Geometry: final body of the model. Coordinates: model frame, mm. Face numbers are marked on the shaded views. Round coordinates to 2 decimals unless told otherwise and drop trailing zeros. Write each loop counter-clockwise with the first axis right and the second up, starting at its lowest first coordinate (ties: lowest second). Pieces come first, ordered by that corner, then holes. Notation, with made-up numbers: M 51,-1 L 79,-1 A12 ccw 79,5 Z; hole C 86,58 d2. An arc over 180 degrees is marked long. Answer as CSV lines item,"result". Start each with the question number.
Q1. First-contact query: pin 1 (5 mm diameter, centred on x = 6.5, y = 4.5, fed in from +Z); pin 2 (2 mm diameter, centred on x = -8, z = 3.5, fed in from +Y); pin 3 (1 mm diameter, centred on x = 11, z = 2, fed in from -Y). Flat tips, straight axial feed; report the tip coordinate or a pass-through.
Q2. Section query A-A on z = 3.25. Output: boundary loops of the cut face in (x, y).
Q3. Section query B-B on x = -9. Output: boundary loops of the cut face in (y, z).
Q4. Ray query, probe 1 along Y at (x, z) = (3.5, 1.2); probe 2 along X at (y, z) = (1.5, 0.55); probe 3 along Z at (x, y) = (9, -1). Return the intervals inside material, ascending.
Q5. Mould query, pull axis X, two halves, no side actions, for the marked faces 1, 2, 3 and 4. Classes: pulls with the +X half, pulls with the -X half, needs draft (parallel to the pull), parting line crosses it, or undercut.
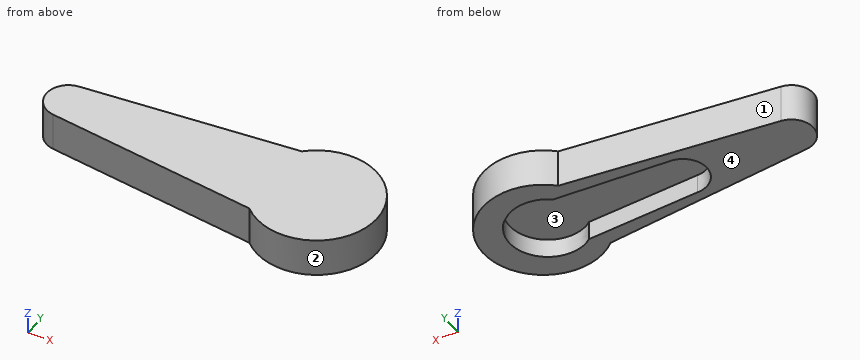
```python
from build123d import *

# Parameters (mm, degrees)
BOSS_EXTRUDE6_DEPTH = 4
CUT_EXTRUDE1_DEPTH  = 2


with BuildPart() as part:
    # Sketch2 → Boss-Extrude6 (new body)
    with BuildSketch(Plane.XY):
        with BuildLine():
            Line((7.936945185, 4.607509822), (-13.764834635, 2.265131203))
            ThreePointArc((-13.764834635, 2.265131203), (-15.798635322, 0), (-13.764834635, -2.265131203))
            Line((-13.764834635, -2.265131203), (7.936945185, -4.607509822))
            ThreePointArc((7.936945185, -4.607509822), (18.479455181, 0), (7.936945185, 4.607509822))
        make_face()
    extrude(amount=BOSS_EXTRUDE6_DEPTH)

    # Sketch1 → Cut-Extrude1 (cut)
    with BuildSketch(Plane.XY):
        with BuildLine():
            Line((-2.308259951, 2.498066053), (9.375044145, 3.190055955))
            add(Edge.make_bspline(
                [(9.375044145, 3.190055955), (9.743762717, 3.535051607), (10.542113364, 3.885379294), (11.739855888, 4.053778423), (12.781606273, 3.904003548), (13.647647588, 3.58835165), (14.172524986, 3.123610305), (14.749448402, 2.727996587), (15.239395752, 2.01553181), (15.653528757, 1.050879588), (15.788992815, -0.000691818), (15.651665108, -1.048112313), (15.246850359, -2.025217286), (14.603250264, -2.863967716), (13.764299096, -3.507779486), (12.787785525, -3.91194775), (11.73820132, -4.051651269), (10.542857019, -3.886335356), (9.743600409, -3.534842939), (9.375044145, -3.190055955)],
                knots=[0, 0, 0, 0, 0.085136877, 0.144403023, 0.203669169, 0.262935434, 0.297502717, 0.322201499, 0.3814676, 0.440733879, 0.5, 0.559266121, 0.6185324, 0.677798501, 0.737064566, 0.796330831, 0.855596977, 0.914863123, 1, 1, 1, 1], degree=3))
            Line((9.375044145, -3.190055955), (-2.308259951, -2.498066053))
            add(Edge.make_bspline(
                [(-2.308259951, -2.498066053), (-2.730270965, -2.498681523), (-3.365255191, -2.317767142), (-4.051947117, -1.791219452), (-4.45450445, -1.266528616), (-4.707556493, -0.655614107), (-4.793872131, 0), (-4.707556493, 0.655614107), (-4.45450445, 1.266528616), (-4.051947117, 1.791219452), (-3.365255191, 2.317767142), (-2.730270965, 2.498681523), (-2.308259951, 2.498066053)],
                knots=[0, 0, 0, 0, 0.162547316, 0.2469105, 0.331273485, 0.415637006, 0.5, 0.584362994, 0.668726515, 0.7530895, 0.837452684, 1, 1, 1, 1], degree=3))
        make_face()
    extrude(amount=CUT_EXTRUDE1_DEPTH, mode=Mode.SUBTRACT)


solid = part.part
```
Entries:
1,pin 1,"stops at z = 4"
1,pin 2,"stops at y = 3"
1,pin 3,"stops at y = -6.24"
2,outline,"M -13.76,-2.27 L 7.94,-4.61 A6.28 ccw long 7.94,4.61 L -13.76,2.27 A2.28 ccw Z"
3,outline,"M -2.78,0 L 2.78,0 L 2.78,4 L -2.78,4 Z"
4,probe 1,"y = -4.13 to -2.84, 2.84 to 4.13"
4,probe 2,"x = -15.24 to -4.27, 15.45 to 18.3"
4,probe 3,"z = 2 to 4"
5,face 1,"pulls with the -X half"
5,face 2,"parting line crosses it"
5,face 3,"undercut"
5,face 4,"needs draft"
